Design review of the part built by this model. Coordinates are the model's own, in mm. Give positions to 0.01 mm unless a question says otherwise; leave off trailing zeros. Write each loop counter-clockwise with the first axis right and the second up, starting at its lowest first coordinate (ties: lowest second). Pieces come first, ordered by that corner, then holes. Notation, with made-up numbers: (-6.75, 87) -> (14.25, 87) arc R21 ccw to (14.25, 96) -> close; hole circle Ø11 at (5, 50). An arc over 180 degrees is marked (long way). Use CSV: the item, a comma, the result in double quotes.
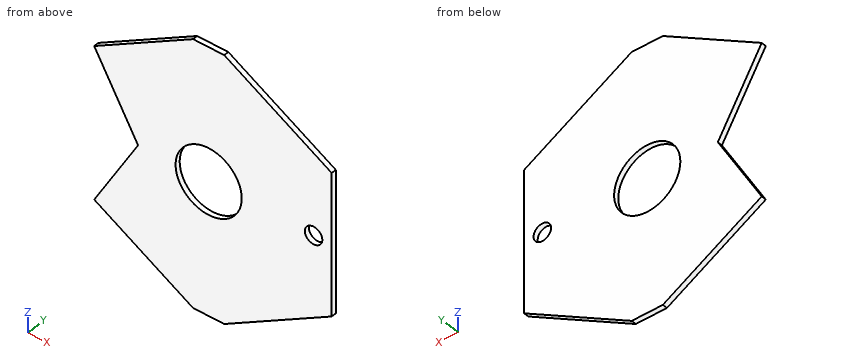
Autodesk Inventor part; units mm, degrees
ref_plane "YZ Plane" through (0, 0, 0) normal (1, 0, 0) x (0, 1, 0)
ref_plane "XZ Plane" through (0, 0, 0) normal (0, 1, 0) x (-1, 0, 0)
ref_plane "XY Plane" through (0, 0, 0) normal (0, 0, 1) x (1, 0, 0)
sketch "Sketch1" plane through (0, 0, 0) normal (0, 1, 0) x (-1, 0, 0)
  circle A0 centre (0, 0) radius 6.625
  line L0 (0, -28.4345) -> (-24.625, -14.2173)
  line L1 (-24.625, -14.2173) -> (-24.625, 14.2173)
  line L2 (-24.625, 14.2173) -> (0, 28.4345)
  line L3 (0, 28.4345) -> (24.625, 14.2173)
  line L4 (24.625, 14.2173) -> (24.625, -14.2173)
  line L5 (24.625, -14.2173) -> (0, -28.4345)
  line L6 (22.9063, 15.2096) -> (14.125, 0)
  line L7 (14.125, 0) -> (22.9062, -15.2096)
  line L8 (14.125, 0) -> (24.625, 0)
  line L9 (3.1177, 26.6345) -> (-3.1177, 26.6345)
  line L10 (3.1177, -26.6345) -> (-3.1177, -26.6345)
  circle A1 centre (-21, 0) radius 1.75
  line L11 (0, 0) -> (-21, 0)
  dimension "d0" = 13.25
  dimension "d1" = 49.25
  dimension "d4" = 120
  dimension "d5" = 120
  dimension "d6" = 10.5
  dimension "d7" = 24.625
  dimension "d8" = 1.8
  dimension "d9" = 1.8
  dimension "d10" = 3.5
  dimension "d11" = 21
extrude "Extrusion1" add sketch "Sketch1" along normal blind 1 contours A1 | L0 L1 L2 L9 L3 L6 L7 L5 L10
extrude "Extrusion2" cut sketch "Sketch1" along normal through all contours A1
properties part number "PCB"
(1) Take a section at B-B (y = 0.8). State how many separate pieces and enclosed holes the cut face has, then the cut area to 3 significant figures.
Established:
separate pieces,"1"
enclosed holes,"2"
area,"1,760 mm2"
(2) For line 1 along X through (y, z) = (0.6, 0) (3 decimals); line 2 along Z through (x, y) = (21, 0.35); line 3 along X through (y, z) = (0.6, -6) (3 decimals), list the stretches that pass through material, from the lowest coordinate up. Write a range as [from, to].
Established:
line 1,"x = [-14.125, -6.625], [6.625, 19.25], [22.75, 24.625]"
line 2,"z = [-16.31, -1.75], [1.75, 16.31]"
line 3,"x = [-17.589, -2.809], [2.809, 24.625]"
(3) Take a section at D-D (x = -11). Write out the cut boundary in (y, z), then the cut area to 3 significant figures.
Established:
outline,"(0, -22.08) -> (1, -22.08) -> (1, 22.08) -> (0, 22.08) -> close"
area,"44.2 mm2"
(4) Take a section at A-A (x = 0). Write out the cut boundary in (y, z) (1 decimal).
Established:
outline,"(0, -26.6) -> (1, -26.6) -> (1, -6.6) -> (0, -6.6) -> close; (0, 6.6) -> (1, 6.6) -> (1, 26.6) -> (0, 26.6) -> close"
(5) Take a section at C-C (z = -2.5). Write out the cut boundary in (x, y) (3 decimals), then the cut area to 3 significant figures.
Established:
outline,"(-15.568, 0) -> (-6.135, 0) -> (-6.135, 1) -> (-15.568, 1) -> close; (6.135, 0) -> (24.625, 0) -> (24.625, 1) -> (6.135, 1) -> close"
area,"27.9 mm2"
